from build123d import *

# Parameters (mm, degrees)
EXTRUDE_1_DEPTH      = 31
EXTRUDE_1_DEPTH_BACK = 31
SKETCH_2_R           = 21
EXTRUDE_2_DEPTH      = 34
EXTRUDE_3_DEPTH      = 8
EXTRUDE_4_DEPTH      = 8
EXTRUDE_5_DEPTH      = 5
EXTRUDE_5_DEPTH_BACK = 5
SKETCH_6_R           = 8
CUT_EXTRUDE_1_DEPTH  = 7
SKETCH_7_R           = 15
CUT_EXTRUDE_2_DEPTH  = 28.0000001
SKETCH_8_R           = 7
CUT_EXTRUDE_3_DEPTH  = 63.0000001
SKETCH_9_R           = 3
CUT_EXTRUDE_4_DEPTH  = 9.0000001


with BuildPart() as part:
    # Sketch 1 → Extrude 1 (new body, two sides)
    with BuildSketch(Plane.XY) as extrude_1_sk:
        with BuildLine():
            Line((-14, 0), (14, 0))
            ThreePointArc((14, 0), (0, 14), (-14, 0))
        make_face()
    extrude(amount=EXTRUDE_1_DEPTH)
    extrude(extrude_1_sk.sketch, amount=-EXTRUDE_1_DEPTH_BACK)

    # Sketch 2 → Extrude 2 (add)
    with BuildSketch(Plane(origin=(0, 0, 0), x_dir=(1, 0, 0), z_dir=(0, 1, 0))):
        Circle(SKETCH_2_R)
    extrude(amount=EXTRUDE_2_DEPTH)

    # Sketch 3 → Extrude 3 (add)
    with BuildSketch(Plane(origin=(0, 0, 0), x_dir=(1, 0, 0), z_dir=(0, 1, 0))):
        with BuildLine():
            Line((0, 25), (0, -25))
            Line((0, -25), (-18, -25))
            Line((-18, -25), (-45.582150825, -5.730583929))
            ThreePointArc((-45.582150825, -5.730583929), (-47.97254676, 0.662191934), (-44.560227187, 6.572999924))
            Line((-44.560227187, 6.572999924), (-18, 25))
            Line((-18, 25), (0, 25))
        make_face()
    extrude(amount=EXTRUDE_3_DEPTH)

    # Sketch 4 → Extrude 4 (add)
    with BuildSketch(Plane(origin=(0, 0, 0), x_dir=(1, 0, 0), z_dir=(0, 1, 0))):
        with BuildLine():
            Line((0, -25), (0, 25))
            Line((0, 25), (22, 25))
            ThreePointArc((22, 25), (27.656854249, 22.656854249), (30, 17))
            Line((30, 17), (30, -17))
            ThreePointArc((30, -17), (27.656854249, -22.656854249), (22, -25))
            Line((22, -25), (0, -25))
        make_face()
    extrude(amount=EXTRUDE_4_DEPTH)

    # Sketch 5 → Extrude 5 (add, two sides)
    with BuildSketch(Plane.XY) as extrude_5_sk:
        Polygon((-16.636065675, 8), (-35, 8), (-26, 18), (-16.636065675, 18), align=None)
    extrude(amount=EXTRUDE_5_DEPTH)
    extrude(extrude_5_sk.sketch, amount=-EXTRUDE_5_DEPTH_BACK)

    # Sketch 6 → Cut-Extrude 1 (cut)
    with BuildSketch(Plane(origin=(0, 34, 0), x_dir=(1, 0, 0), z_dir=(0, 1, 0))):
        Circle(SKETCH_6_R)
    extrude(amount=-CUT_EXTRUDE_1_DEPTH, mode=Mode.SUBTRACT)

    # Sketch 7 → Cut-Extrude 2 (cut, through all)
    with BuildSketch(Plane(origin=(0, 27, 0), x_dir=(1, 0, 0), z_dir=(0, 1, 0))):
        Circle(SKETCH_7_R)
    extrude(amount=-CUT_EXTRUDE_2_DEPTH, mode=Mode.SUBTRACT)

    # Sketch 8 → Cut-Extrude 3 (cut, through all)
    with BuildSketch(Plane.XY.offset(31)):
        Circle(SKETCH_8_R)
    extrude(amount=-CUT_EXTRUDE_3_DEPTH, mode=Mode.SUBTRACT)

    # Sketch 9 → Cut-Extrude 4 (cut, through all)
    with BuildSketch(Plane(origin=(0, 8, 0), x_dir=(1, 0, 0), z_dir=(0, 1, 0))):
        with Locations((-40, 0)):
            Circle(SKETCH_9_R)
        with Locations((20, 16)):
            Circle(SKETCH_9_R)
        with Locations((20, -16)):
            Circle(SKETCH_9_R)
    extrude(amount=-CUT_EXTRUDE_4_DEPTH, mode=Mode.SUBTRACT)


solid = part.part
Design review of the part built by this model. Coordinates are the model's own, in mm. A direction names the side the tool comes from. Round coordinates to 2 decimals unless told otherwise and drop trailing zeros. Order: outer loops, then holes, each group sorted by start corner. A loop starts at its lowest first (then second) coordinate and runs counter-clockwise, first axis right, second up.
1) Draft analysis for pull direction Z (two halves, no side actions). For faces 6 (the cylindrical face through (17.6, 4.1, -14.2)), 7 (the flat face through (18, 0, 0)), 8 (the flat face through (18, 4, 25)), state which applies: released by +Z, released by -Z, zero draft, split by the parting line, or undercut.
The answers:
face 6: undercut
face 7: zero draft
face 8: released by +Z
2) Consider section C-C (x = 20). State the section outline as (y, z) points, plus the area to 3 significant figures.
The answers:
outline: (0, -25) - (8, -25) - (8, -19) - (0, -19) - close; (0, -13) - (8, -13) - (8, -6.4) - (34, -6.4) - (34, 6.4) - (8, 6.4) - (8, 13) - (0, 13) - close; (0, 19) - (8, 19) - (8, 25) - (0, 25) - close
area: 637 mm2
3) Consider section B-B (y = 6). State the section outline as (x, z) points.
The answers:
outline: (-45.58, 5.73) arc R8 ccw to (-44.56, -6.57) - (-18, -25) - (-12.65, -25) - (-12.65, -31) - (-3.61, -31) - (-3.61, -14.56) arc R15 cw to (-3.61, 14.56) - (-3.61, 31) - (-12.65, 31) - (-12.65, 25) - (-18, 25) - close; (3.61, -31) - (12.65, -31) - (12.65, -25) - (22, -25) arc R8 ccw to (30, -17) - (30, 17) arc R8 ccw to (22, 25) - (12.65, 25) - (12.65, 31) - (3.61, 31) - (3.61, 14.56) arc R15 cw to (3.61, -14.56) - close; hole circle Ø6 at (-40, 0); hole circle Ø6 at (20, -16); hole circle Ø6 at (20, 16)
4) Consider section D-D (x = -1.5). State the section outline as (y, z) points.
The answers:
outline: (6.84, -31) - (13.92, -31) - (13.92, -20.95) - (34, -20.95) - (34, -7.86) - (27, -7.86) - (27, -14.92) - (6.84, -14.92) - close; (6.84, 14.92) - (27, 14.92) - (27, 7.86) - (34, 7.86) - (34, 20.95) - (13.92, 20.95) - (13.92, 31) - (6.84, 31) - close
5) Consider section A-A (z = 0). State the section outline as (x, y) points.
The answers:
outline: (-48, 0) - (-43, 0) - (-43, 8) - (-48, 8) - close; (-37, 0) - (-15, 0) - (-15, 27) - (-8, 27) - (-8, 34) - (-21, 34) - (-21, 18) - (-26, 18) - (-35, 8) - (-37, 8) - close; (8, 27) - (15, 27) - (15, 0) - (30, 0) - (30, 8) - (21, 8) - (21, 34) - (8, 34) - close
6) Machinability: for faces 1 (the cylindrical face through (14.307, 13.689, -4.506)), 2 (the flat face through (-26, 12, -5)), 3 (the cylindrical face through (0, 14, 26)), 4 (the cylindrical face through (20.03, 20.82, -6.31)), 5 (the flat face through (-26, 12, 5)), which of the approach directions +Z, -Z, +X, -X, +Y, -Y give a long, thin tool a straight path to every point of the face, cutting with its end or side? Answer none if there is none.
The answers:
face 1: -Y
face 2: -Z, -X, +Y
face 3: +Z, +Y
face 4: +Y
face 5: +Z, -X, +Y
7) For L1, parallel to X at y = 5, z = 0; L2, parallel to X at y = 32, z = 0; L3, parallel to Z at x = 20, y = 3, list the stretches that pass through material, from the lowest coordinate up.
The answers:
L1: x = -48 to -43, -37 to -15, 15 to 30
L2: x = -21 to -8, 8 to 21
L3: z = -25 to -19, -13 to 13, 19 to 25
8) Clearance check with flat-ended pins moving along their axes: pin 1 Ø5 at (x, y) = (-28.5, 14) entering from +Z; pin 2 Ø2 at (x, y) = (-15.5, 2) entering from +Z; pin 3 Ø5 at (x, z) = (20, -16) entering from +Y; pin 4 Ø5 at (y, z) = (22.5, 4.5) entering from -X. State where each tip first meets the part, or that it passes through.
The answers:
pin 1: stops at z = 5
pin 2: stops at z = 25
pin 3: passes through
pin 4: stops at x = -20.9
